Could you check a few things on this model? Use its own coordinates, in mm. A direction names the side the tool comes from. Round coordinates to 2 decimals unless told otherwise and drop trailing zeros. Loops run counter-clockwise (first coordinate to the right, second up) from the corner with the lowest first, then second, coordinate; pieces in that order, holes last. Notation, with made-up numbers: M 22,30 L 69,30 A22 cw 69,56 Z; hole C -20.75,26 d11. An arc over 180 degrees is marked long. One line per item, written item: value. Start each with the question number.
Q1. Imagine slicing it at C-C (y = 4). Please give me the cut outline in (x, z).
Q2. Imagine slicing it at A-A (z = -1). Please give me the cut outline in (x, y) (3 decimals).
Q3. Imagine slicing it at D-D (x = 13.5). Please give me the cut outline in (y, z) (1 decimal), then the cut area to 3 significant figures.
Q4. Thinking about a two-plate mould opening in Z: for faces 1 (the face through (-23, 7, 31.102)), 2 (the face through (0, 15, -37.782)), 3 (the face through (-21.26, 7, 33)), which applies, released by +Z, released by -Z, zero draft, split by the parting line, or undercut?
Q5. Which directions (+Z, -Z, +X, -X, +Y, -Y) give clear straight access to the entire face, cutting with the end or side of a thin tool? Please do faces 4 (the face through (-11.43, 1, -1)), 5 (the face through (21.26, 7, -33)), 6 (the face through (-23, 7, -31.102)).
Q6. I'm going to push flat-ended pins straight in: pin 1 Ø2 at (x, z) = (-23.5, -33.5) entering from +Y; pin 2 Ø2 at (x, y) = (10.5, 19) entering from +Z; pin 3 Ø1 at (x, z) = (-15, 15) entering from +Y. Where does each tip first touch, or does it pass through?
Q7. Imagine slicing it at B-B (x = -10.5). Please give me the cut outline in (y, z) (1 decimal), then the cut area to 3 significant figures.
Q8. Please list where these lines run through material, in increasing order: line 1 along X through (y, z) = (16.5, 31.5); line 2 along Y through (x, z) = (0.5, -1.5); line 3 along Z through (x, y) = (-3.5, 27).
from build123d import *

# Parameters (mm, degrees)
SKETCH1_W           = 50.8
SKETCH1_H           = 70.485
BOSS_EXTRUDE1_DEPTH = 2.54
BOSS_EXTRUDE2_DEPTH = 31.115
SKETCH6_W           = 4.1402
SKETCH6_H           = 4.1402
BOSS_EXTRUDE3_DEPTH = 8.128
SKETCH8_W           = 9.398
SKETCH8_H           = 24.13
CUT_EXTRUDE2_DEPTH  = 3.54


with BuildPart() as part:
    # Sketch1 → Boss-Extrude1 (new body)
    with BuildSketch(Plane(origin=(0, 0, 0), x_dir=(1, 0, 0), z_dir=(0, 1, 0))):
        Rectangle(SKETCH1_W, SKETCH1_H)
    extrude(amount=BOSS_EXTRUDE1_DEPTH)

    # Sketch5 → Boss-Extrude2 (add)
    with BuildSketch(Plane(origin=(0, 0, 0), x_dir=(1, 0, 0), z_dir=(0, 1, 0))):
        Polygon((27.94, -35.2425), (27.94, 37.7825), (-27.94, 37.7825), (-27.94, -35.2425), (-25.4, -35.2425), (-25.4, 35.2425), (25.4, 35.2425), (25.4, -35.2425), align=None)
    extrude(amount=BOSS_EXTRUDE2_DEPTH)

    # Sketch6 → Boss-Extrude3 (add)
    with BuildSketch(Plane(origin=(0, 2.54, 0), x_dir=(1, 0, 0), z_dir=(0, 1, 0))):
        with Locations((-23.3299, 33.1724)):
            Rectangle(SKETCH6_W, SKETCH6_H)
        with Locations((23.3299, 33.1724)):
            Rectangle(SKETCH6_W, SKETCH6_H)
        with Locations((23.3299, -33.1724)):
            Rectangle(SKETCH6_W, SKETCH6_H)
        with Locations((-23.3299, -33.1724)):
            Rectangle(SKETCH6_W, SKETCH6_H)
    extrude(amount=BOSS_EXTRUDE3_DEPTH)

    # Sketch8 → Cut-Extrude2 (cut, through all)
    with BuildSketch(Plane(origin=(0, 2.54, 0), x_dir=(1, 0, 0), z_dir=(0, 1, 0))):
        with Locations((-6.731, 0.8255)):
            Rectangle(SKETCH8_W, SKETCH8_H)
    extrude(amount=-CUT_EXTRUDE2_DEPTH, mode=Mode.SUBTRACT)


solid = part.part
Report:
1. outline: M -27.94,-37.78 L 27.94,-37.78 L 27.94,35.24 L 21.26,35.24 L 21.26,31.1 L 25.4,31.1 L 25.4,-31.1 L 21.26,-31.1 L 21.26,-35.24 L -21.26,-35.24 L -21.26,-31.1 L -25.4,-31.1 L -25.4,31.1 L -21.26,31.1 L -21.26,35.24 L -27.94,35.24 Z
2. outline: M -27.94,0 L -11.43,0 L -11.43,2.54 L -25.4,2.54 L -25.4,31.115 L -27.94,31.115 Z; M -2.032,0 L 27.94,0 L 27.94,31.115 L 25.4,31.115 L 25.4,2.54 L -2.032,2.54 Z
3. outline: M 0,-37.8 L 31.1,-37.8 L 31.1,-35.2 L 2.5,-35.2 L 2.5,35.2 L 0,35.2 Z
3. area: 258 mm²
4. face 1: undercut
4. face 2: released by -Z
4. face 3: zero draft
5. face 4: +Y, -Y
5. face 5: +Z, +Y
5. face 6: +Y
6. pin 1: stops at y = 10.67
6. pin 2: stops at z = -35.24
6. pin 3: stops at y = 2.54
7. outline: M 0,-37.8 L 31.1,-37.8 L 31.1,-35.2 L 2.5,-35.2 L 2.5,-12.9 L 0,-12.9 Z; M 0,11.2 L 2.5,11.2 L 2.5,35.2 L 0,35.2 Z
7. area: 197 mm²
8. line 1: x = -27.94 to -25.4, 25.4 to 27.94
8. line 2: y = 0 to 2.54
8. line 3: z = -37.78 to -35.24
